```python
from build123d import *
from build123d.topology import SkipClean

# Parameters (mm, degrees)
EXTRUDE_2_DEPTH                = 5
EXTRUDE_2_DEPTH_BACK           = 5
SKETCH_1_R                     = 34
EXTRUDE_3_DEPTH                = 8
EXTRUDE_START                  = -3
SKETCH_3_R                     = 46.25
SKETCH_3_R_2                   = 34
EXTRUDE_4_DEPTH                = 3
EXTRUDE_5_DEPTH                = 27.3
EXTRUDE_5_DEPTH_BACK           = 3
SKETCH_4_R                     = 51.25
SKETCH_4_R_2                   = 46.25
HOLE_WIZARD_M3_5_1_D           = 2.9
HOLE_WIZARD_M3_5_1_CSINK_D     = 3.55
HOLE_WIZARD_M3_5_1_CSINK_ANGLE = 90
PATTERN_CIRCULAR_2_COUNT       = 8
EXTRUDE_6_DEPTH                = 10
EXTRUDE_6_DEPTH_BACK           = 4
SKETCH_11_R                    = 15
PATTERN_CIRCULAR_3_COUNT       = 4


with BuildPart() as part:
    # 草图1 → 凸台-拉伸2 (new, two sides: drawn at the far end of the back side and taken through both)
    with BuildSketch(Plane(origin=(0, 0, 0), x_dir=(1, 0, 0), z_dir=(0, 1, 0)).offset(-EXTRUDE_2_DEPTH_BACK)):
        with Locations(Location((0, 0, 0), (0, 0, 270))):
            Circle(SKETCH_1_R)
    extrude(amount=EXTRUDE_2_DEPTH + EXTRUDE_2_DEPTH_BACK)

    # 草图2 → 凸台-拉伸3 (add)
    with SkipClean():  # the faces are left unmerged after this step: merging them gives an invalid solid
        with BuildSketch(Plane(origin=(0, 5, 0), x_dir=(1, 0, 0), z_dir=(0, 1, 0))):
            with BuildLine():
                Line((-34, 0), (-29, 0))
                ThreePointArc((-29, 0), (-25.11473671, 14.5), (-14.5, 25.11473671))
                Line((-14.5, 25.11473671), (-17, 29.444863729))
                ThreePointArc((-17, 29.444863729), (-29.444863729, 17), (-34, 0))
            make_face()
            with BuildLine():
                Line((29, 0), (34, 0))
                ThreePointArc((34, 0), (29.444863729, -17), (17, -29.444863729))
                Line((17, -29.444863729), (14.5, -25.11473671))
                ThreePointArc((14.5, -25.11473671), (25.11473671, -14.5), (29, 0))
            make_face()
        extrude(amount=EXTRUDE_3_DEPTH)

    # 草图3 → 凸台-拉伸4 (add)
    with SkipClean():  # the faces are left unmerged after this step: merging them gives an invalid solid
        with BuildSketch(Plane(origin=(0, 13, 0), x_dir=(1, 0, 0), z_dir=(0, 1, 0)).offset(EXTRUDE_START)):
            with Locations(Location((0, 0, 0), (0, 0, 270))):
                Circle(SKETCH_3_R)
            with Locations(Location((0, 0, 0), (0, 0, 270))):
                Circle(SKETCH_3_R_2, mode=Mode.SUBTRACT)
        extrude(amount=EXTRUDE_4_DEPTH)

    # 草图4 → 凸台-拉伸5 (add, two sides: drawn at the far end of the back side and taken through both)
    with SkipClean():  # the faces are left unmerged after this step: merging them gives an invalid solid
        with BuildSketch(Plane(origin=(0, 13, 0), x_dir=(1, 0, 0), z_dir=(0, 1, 0)).offset(-EXTRUDE_5_DEPTH_BACK)):
            with Locations(Location((0, 0, 0), (0, 0, 270))):
                Circle(SKETCH_4_R)
            with Locations(Location((0, 0, 0), (0, 0, 270))):
                Circle(SKETCH_4_R_2, mode=Mode.SUBTRACT)
        extrude(amount=EXTRUDE_5_DEPTH + EXTRUDE_5_DEPTH_BACK)

    # M3.5 螺纹孔1 (through all)
    with Locations(Plane.XZ.offset(-10)):
        with Locations((36.806079661, 21.25)):
            hole_wizard_m3_5_1 = CounterSinkHole(HOLE_WIZARD_M3_5_1_D / 2, HOLE_WIZARD_M3_5_1_CSINK_D / 2, counter_sink_angle=HOLE_WIZARD_M3_5_1_CSINK_ANGLE)

    # 阵列(圆周)2: M3.5 螺纹孔1 ×8 about axis
    with SkipClean():  # the faces are left unmerged after this step: merging them gives an invalid solid
        pattern_circular_2_axis = Axis((0, 0, 0), (0, 1, 0))
        for i in range(1, PATTERN_CIRCULAR_2_COUNT):
            add(hole_wizard_m3_5_1.rotate(pattern_circular_2_axis, i * 360 / PATTERN_CIRCULAR_2_COUNT), mode=Mode.SUBTRACT)

    # 草图11 → 凸台-拉伸6 (add, two sides: drawn at the far end of the back side and taken through both)
    with SkipClean():  # the faces are left unmerged after this step: merging them gives an invalid solid
        with BuildSketch(Plane(origin=(51.25, 0, 0), x_dir=(0, 0, -1), z_dir=(1, 0, 0)).offset(-EXTRUDE_6_DEPTH_BACK)):
            with Locations((0, 25)):
                Circle(SKETCH_11_R)
        extrude(amount=EXTRUDE_6_DEPTH + EXTRUDE_6_DEPTH_BACK)

    # 草图14 → M4 螺纹孔1 (revolve, cut)
    with SkipClean():  # the faces are left unmerged after this step: merging them gives an invalid solid
        with BuildSketch(Plane(origin=(61.25, 33, 0), x_dir=(0, 0, -1), z_dir=(0, 1, 0))):
            Polygon((0, 0), (0, 11.091420021), (1.65, 10.1), (1.65, 0.375), (2.025, 0), align=None)
        hole_wizard_m4_1 = revolve(axis=Axis((67.6, 33, 0), (-1, 0, 0)), mode=Mode.SUBTRACT)

    # 阵列(圆周)3: M4 螺纹孔1 ×4 about axis
    with SkipClean():  # the faces are left unmerged after this step: merging them gives an invalid solid
        pattern_circular_3_axis = Axis((0, 24.851493468, 0), (1, 0, 0))
        for i in range(1, PATTERN_CIRCULAR_3_COUNT):
            add(hole_wizard_m4_1.rotate(pattern_circular_3_axis, i * 360 / PATTERN_CIRCULAR_3_COUNT), mode=Mode.SUBTRACT)


solid = part.part
```
Part model, mm, in its own coordinate system. A direction names the side the tool comes from. Coordinates: 2 decimals unless noted, no trailing zeros. Write each loop counter-clockwise with the first axis right and the second up, starting at its lowest first coordinate (ties: lowest second). Pieces come first, ordered by that corner, then holes.
Item 1: Slice it at D-D (y = 2). Write the cut outline in (x, z).
Item 2: Mould opens along Z. For faces 4 (the face through (-17.43, 11.479, 29.192)), 5 (the face through (0, -5, 0)), 6 (the face through (15.768, 8.944, 27.31)) say: released by +Z, released by -Z, zero draft, split by the parting line, or undercut.
Item 3: Slice it at C-C (z = -21.25). Write the cut outline in (x, y) (3 decimals).
Item 4: Slice it at A-A (y = 8.5). Write the cut outline in (x, z).
Item 5: Slice it at B-B (x = 0). Write the cut outline in (y, z).
Item 6: Which spindle directions (+Z, -Z, +X, -X, +Y, -Y) get a long thin tool onto all of the face, cutting with end or side? Do faces 1 (the face through (56.081, 15.092, -0.358)), 2 (the face through (-37.12, 11.681, -19.834)), 3 (the face through (31, 9, 0)). Say none if no direction does.
Item 7: Pin check, flat tips, straight feed: pin 1 (8 mm diameter, centred on x = 11, z = -8, fed in from +Y); pin 2 (2 mm diameter, centred on y = 33, z = 0, fed in from +X); pin 3 (1.5 mm diameter, centred on x = -15, y = 7, fed in from -Z); pin 4 (2.5 mm diameter, centred on x = 36.81, z = 21.25, fed in from -Y). Stop position of each tip, or through.
Item 8: Probe line 1 (X direction, y = 11.5, z = 11.5); line 2 (X direction, y = 35, z = 1); line 3 (Y direction, x = 20, z = -19.5). List the from-to ranges inside material, lowest first.
Results found:
1. outline: circle Ø68 at (0, 0)
2. face 4: undercut
2. face 5: zero draft
2. face 6: undercut
3. outline: (-46.637, 10) - (-38.581, 10) - (-38.256, 10.325) - (-38.256, 13) - (-41.079, 13) - (-41.079, 40.3) - (-46.637, 40.3) - close; (-35.356, 10.325) - (-35.031, 10) - (-26.541, 10) - (-26.541, -5) - (26.541, -5) - (26.541, 5) - (-19.734, 5) - (-19.734, 13) - (-35.356, 13) - close; (26.541, 10) - (46.637, 10) - (46.637, 40.3) - (41.079, 40.3) - (41.079, 13) - (26.541, 13) - close
4. outline: (-34, 0) arc R34 ccw to (-17, -29.44) - (-14.5, -25.11) arc R29 cw to (-29, 0) - close; (14.5, 25.11) arc R29 cw to (29, 0) - (34, 0) arc R34 ccw to (17, 29.44) - close
5. outline: (-5, -34) - (5, -34) - (5, 34) - (-5, 34) - close; (10, -51.25) - (40.3, -51.25) - (40.3, -46.25) - (13, -46.25) - (13, -34) - (10, -34) - close; (10, 34) - (13, 34) - (13, 46.25) - (40.3, 46.25) - (40.3, 51.25) - (10, 51.25) - close
6. face 1: +X
6. face 2: +Y, -Y
6. face 3: +Y
7. pin 1: stops at y = 5
7. pin 2: stops at x = 50.76
7. pin 3: stops at z = -27.28
7. pin 4: passes through
8. line 1: x = -49.94 to -42.41, -39.69 to -32, 26.62 to 49.94
8. line 2: x = -51.24 to -46.24, 46.24 to 61.25
8. line 3: y = -5 to 5
